For this review, take the finished solid that the model builds, in its own axes (mm). A direction names the side the tool comes from. Coordinates: 2 decimals unless noted, no trailing zeros. Order: outer loops, then holes, each group sorted by start corner. A loop starts at its lowest first (then second) coordinate and runs counter-clockwise, first axis right, second up. Notation, with made-up numbers: (71.25, 28) -> (104.25, 28) arc R14 ccw to (104.25, 55) -> close; hole circle Ø10 at (85, 11.5). An arc over 180 degrees is marked (long way). Write item = value, one per line. Start each with the question number.
1) Draft analysis for pull direction X (two halves, no side actions). For faces 6 (the face through (32, 0, 20)), 7 (the face through (0, -19, 0)), 8 (the face through (44, -1, 22)), 9 (the face through (44, -19.556, 20)), state which applies: +X half, -X half, draft (parallel to the pull), parting line (faces both ways), or undercut.
2) Machinability: for faces 1 (the face through (5.25, -1, 19.78)), 2 (the face through (22, -17, -1)), 3 (the face through (26, -10, 23.75)), 4 (the face through (4.794, -10.148, -19.738)), 5 (the face through (44, -19.556, -20)), which of the approach directions +Z, -Z, +X, -X, +Y, -Y give a long, thin tool a straight path to every point of the face, cutting with its end or side? Answer none if there is none.
3) Consider section C-C on x = 32.5. Give the boundary of the cut face in (y, z), and give its area (3 significant figures).
4) Consider section B-B on y = -4. Give the boundary of the cut face in (x, z) (3 decimals), and give its area (3 significant figures).
5) Consider section A-A on z = 21.25. Give the boundary of the cut face in (x, y).
6) Consider section D-D on x = 45. State how many separate pieces and enclosed holes the cut face has, and give its area (3 significant figures).
7) Wall thickness on probe 1 along X at (y, z) = (-5.5, 21.25); probe 2 along X at (y, z) = (-2.25, -21); probe 3 along Z at (x, y) = (36.5, -4): over which ranges is each line inside the solid? List them lowest first. Write a range as [from, to].
8) Insertion check: pin 1 Ø5 at (x, z) = (45.5, -20.5) entering from +Y; pin 2 Ø1.5 at (x, z) = (41.5, 5.5) entering from +Y; pin 3 Ø2 at (x, z) = (5, 21.5) entering from -Y. Each pin has a flat end and moves straight along its axis. Give the tip position at first contact, or say it passes through.
from build123d import *

# Parameters (mm, degrees)
SALIENTE_EXTRUIR1_DEPTH = 22
SALIENTE_EXTRUIR2_DEPTH = 30.7
CORTAR_EXTRUIR2_REACH   = 63.351
CROQUIS4_R              = 1.585
CROQUIS5_W              = 4.32
CROQUIS5_H              = 4.315133256
CROQUIS5_H_2            = 4.32
CORTAR_EXTRUIR3_DEPTH   = 1
CROQUIS6_W              = 4.32
CROQUIS6_H              = 4.32
CORTAR_EXTRUIR4_DEPTH   = 1


with BuildPart() as part:
    # Croquis1 → Saliente-Extruir1 (new body)
    with BuildSketch(Plane(origin=(0, 0, 0), x_dir=(0, 0, -1), z_dir=(1, 0, 0))):
        with BuildLine():
            Line((-23.75, 0), (-18.75, 0))
            ThreePointArc((-18.75, 0), (0, -18.75), (18.75, 0))
            Line((18.75, 0), (23.75, 0))
            Line((23.75, 0), (23.75, -20.555666233))
            Line((23.75, -20.555666233), (-23.75, -20.555666233))
            Line((-23.75, -20.555666233), (-23.75, 0))
        make_face()
    extrude(amount=SALIENTE_EXTRUIR1_DEPTH)

    # Croquis2 → Saliente-Extruir2 (add)
    with BuildSketch(Plane(origin=(22, 0, 0), x_dir=(0, 0, -1), z_dir=(1, 0, 0))):
        with BuildLine():
            Line((16.75, 0), (23.75, 0))
            Line((23.75, 0), (23.75, -20.555666233))
            Line((23.75, -20.555666233), (-23.75, -20.555666233))
            Line((-23.75, -20.555666233), (-23.75, 0))
            Line((-23.75, 0), (-16.75, 0))
            ThreePointArc((-16.75, 0), (0, -16.75), (16.75, 0))
        make_face()
    extrude(amount=SALIENTE_EXTRUIR2_DEPTH)

    # Croquis4 → Cortar-Extruir2 (cut, up to next)
    with BuildSketch(Plane(origin=(0, 0, 0), x_dir=(1, 0, 0), z_dir=(0, 1, 0)), mode=Mode.PRIVATE) as cortar_extruir2_sk1:
        with Locations(Location((4.31807399, 21.25, 0), (0, 0, 270))):
            Circle(CROQUIS4_R)
    cortar_extruir2_tool1 = extrude(cortar_extruir2_sk1.sketch, amount=-CORTAR_EXTRUIR2_REACH, mode=Mode.PRIVATE) & part.part
    # Croquis4 → Cortar-Extruir2 (cut, up to next)
    with BuildSketch(Plane(origin=(0, 0, 0), x_dir=(1, 0, 0), z_dir=(0, 1, 0)), mode=Mode.PRIVATE) as cortar_extruir2_sk2:
        with Locations(Location((45.631200307, 21.25, 0), (0, 0, 270))):
            Circle(CROQUIS4_R)
    cortar_extruir2_tool2 = extrude(cortar_extruir2_sk2.sketch, amount=-CORTAR_EXTRUIR2_REACH, mode=Mode.PRIVATE) & part.part
    cortar_extruir2_1 = cortar_extruir2_tool1.solids().sort_by_distance((4.318074, 0, -21.25))[0]
    add(cortar_extruir2_1, mode=Mode.SUBTRACT)
    cortar_extruir2_2 = cortar_extruir2_tool2.solids().sort_by_distance((45.6312, 0, -21.25))[0]
    add(cortar_extruir2_2, mode=Mode.SUBTRACT)
    cortar_extruir2 = cortar_extruir2_1 + cortar_extruir2_2  # Cortar-Extruir2 as one shape, for the pattern or mirror that repeats it

    # Simetría1: Cortar-Extruir2 across plane
    add(cortar_extruir2.mirror(Plane.XY), mode=Mode.SUBTRACT)

    # Croquis5 → Cortar-Extruir3 (cut)
    with BuildSketch(Plane(origin=(0, 0, 0), x_dir=(1, 0, 0), z_dir=(0, 1, 0))):
        with Locations((4.31807399, -21.25)):
            Rectangle(CROQUIS5_W, CROQUIS5_H)
        with Locations((45.631200307, -21.25)):
            Rectangle(CROQUIS5_W, CROQUIS5_H_2)
    cortar_extruir3 = extrude(amount=-CORTAR_EXTRUIR3_DEPTH, mode=Mode.SUBTRACT)

    # Croquis6 → Cortar-Extruir4 (cut)
    with BuildSketch(Plane.XZ.offset(20.555666233)):
        with Locations((4.31807399, 21.25)):
            Rectangle(CROQUIS6_W, CROQUIS6_H)
        with Locations((45.631200307, 21.25)):
            Rectangle(CROQUIS6_W, CROQUIS6_H)
    cortar_extruir4 = extrude(amount=-CORTAR_EXTRUIR4_DEPTH, mode=Mode.SUBTRACT)

    # Simetría2: Cortar-Extruir3, Cortar-Extruir4 across plane
    add(cortar_extruir3.mirror(Plane.XY), mode=Mode.SUBTRACT)
    add(cortar_extruir4.mirror(Plane.XY), mode=Mode.SUBTRACT)


solid = part.part
Answer sheet:
q1.face_6 = draft
q1.face_7 = -X half
q1.face_8 = undercut
q1.face_9 = undercut
q2.face_1 = +Y
q2.face_2 = -X, +Y
q2.face_3 = +Z, +X, -X, +Y, -Y
q2.face_4 = +Y, -Y
q2.face_5 = -Y
q3.outline = (-20.56, -23.75) -> (0, -23.75) -> (0, -16.75) arc R16.75 cw to (0, 16.75) -> (0, 23.75) -> (-20.56, 23.75) -> close
q3.area = 536 mm2
q4.outline = (0, -23.75) -> (52.7, -23.75) -> (52.7, -16.265) -> (22, -16.265) -> (22, -18.318) -> (0, -18.318) -> close; (0, 18.318) -> (22, 18.318) -> (22, 16.265) -> (52.7, 16.265) -> (52.7, 23.75) -> (0, 23.75) -> close; hole circle Ø3.17 at (4.318, -21.25); hole circle Ø3.17 at (4.318, 21.25); hole circle Ø3.17 at (45.631, -21.25); hole circle Ø3.17 at (45.631, 21.25)
q4.area = 667 mm2
q5.outline = (0, -20.56) -> (2.16, -20.56) -> (2.16, -19.56) -> (2.73, -19.56) -> (2.73, -1) -> (2.16, -1) -> (2.16, 0) -> (0, 0) -> close; (5.9, -19.56) -> (6.48, -19.56) -> (6.48, -20.56) -> (43.47, -20.56) -> (43.47, -19.56) -> (44.05, -19.56) -> (44.05, -1) -> (43.47, -1) -> (43.47, 0) -> (6.48, 0) -> (6.48, -1) -> (5.9, -1) -> close; (47.22, -19.56) -> (47.79, -19.56) -> (47.79, -20.56) -> (52.7, -20.56) -> (52.7, 0) -> (47.79, 0) -> (47.79, -1) -> (47.22, -1) -> close
q6.separate_pieces = 3
q6.enclosed_holes = 0
q6.area = 410 mm2
q7.probe_1 = [0, 2.73], [5.9, 44.05], [47.22, 52.7]
q7.probe_2 = [0, 2.75], [5.88, 44.07], [47.2, 52.7]
q7.probe_3 = [-23.75, -16.27], [16.27, 23.75]
q8.pin_1 = 0
q8.pin_2 = -15.54
q8.pin_3 = -19.56
